The listing builds one solid part. Answer for the finished solid, in the listing's coordinates (mm). A direction names the side the tool comes from. Round coordinates to 2 decimals unless told otherwise and drop trailing zeros. Write each loop counter-clockwise with the first axis right and the second up, starting at its lowest first coordinate (ties: lowest second). Pieces come first, ordered by that corner, then holes.
from build123d import *

# Parameters (mm, degrees)
F1_DEPTH = 6.35
F2_T     = -6.35


with BuildPart() as f1:
    # F0 (on Top) → F1 (new body)
    with BuildSketch(Plane.XY):
        Polygon((38.1, 38.1), (38.1, 76.2), (-38.1, 76.2), (-38.1, 38.1), (-50.8, 38.1), (-50.8, -38.1), (-38.1, -38.1), (-38.1, -76.2), (38.1, -76.2), (38.1, -38.1), (50.8, -38.1), (50.8, 38.1), align=None)
    extrude(amount=F1_DEPTH)

    # F2
    f2_openings = [f1.faces().sort_by_distance(p)[0] for p in [
        (0, 0, 6.35),
        (0, 0, 0),
    ]]
    offset(amount=F2_T, openings=f2_openings, kind=Kind.INTERSECTION)


solid = f1.part
1. Straight lines are drawn through the part: line 1 along X through (y, z) = (-13, 6); line 2 along Y through (x, z) = (-34, 0.75); line 3 along X through (y, z) = (-65.5, 1.5). For each, find the intervals that lie inside material, in ascending order.
Geometry says:
line 1: x = -50.8 to -44.45, 44.45 to 50.8
line 2: y = -76.2 to -31.75, 31.75 to 76.2
line 3: x = -38.1 to -31.75, 31.75 to 38.1
2. Section A-A on y = 34 is taken. Determine the outline of the cut face in (x, z).
Geometry says:
outline: (-50.8, 0) - (-31.75, 0) - (-31.75, 6.35) - (-50.8, 6.35) - close; (31.75, 0) - (50.8, 0) - (50.8, 6.35) - (31.75, 6.35) - close
3. Section C-C on z = 2 is taken. Determine the outline of the cut face in (x, y), plus the area to 3 significant figures.
Geometry says:
outline: (-50.8, -38.1) - (-38.1, -38.1) - (-38.1, -76.2) - (38.1, -76.2) - (38.1, -38.1) - (50.8, -38.1) - (50.8, 38.1) - (38.1, 38.1) - (38.1, 76.2) - (-38.1, 76.2) - (-38.1, 38.1) - (-50.8, 38.1) - close; hole (-44.45, -31.75) - (-31.75, -31.75) - (-31.75, -69.85) - (31.75, -69.85) - (31.75, -31.75) - (44.45, -31.75) - (44.45, 31.75) - (31.75, 31.75) - (31.75, 69.85) - (-31.75, 69.85) - (-31.75, 31.75) - (-44.45, 31.75) - close
area: 3,060 mm2
4. Given pin 1 (1 mm diameter, centred on y = -38.5, z = 1, fed in from +X); pin 2 (3 mm diameter, centred on y = -45.5, z = 3.5, fed in from +X); pin 3 (3 mm diameter, centred on x = -44, z = 3, fed in from +Y); pin 4 (3 mm diameter, centred on y = 65, z = 4, fed in from -X), each flat-ended and moving along its own axis, determine where each tip first touches the part or whether it passes through.
Geometry says:
pin 1: stops at x = 50.8
pin 2: stops at x = 38.1
pin 3: stops at y = 38.1
pin 4: stops at x = -38.1
5. Section B-B on x = 8 is taken. Determine the outline of the cut face in (y, z).
Geometry says:
outline: (-76.2, 0) - (-69.85, 0) - (-69.85, 6.35) - (-76.2, 6.35) - close; (69.85, 0) - (76.2, 0) - (76.2, 6.35) - (69.85, 6.35) - close
6. A tool of negligible diameter and unlimited length cuts with its end or side. For faces 1 (the face through (38.1, 57, 3)), 2 (the face through (-45, -38.1, 3)), 3 (the face through (38.1, -57, 3)), from which of +Z, -Z, +X, -X, +Y, -Y can it reach the whole face along a straight path? Write none if from no direction.
Geometry says:
face 1: +Z, -Z, +X, +Y
face 2: +Z, -Z, -X, -Y
face 3: +Z, -Z, +X, -Y
7. For a pull along X with two mould halves and no side action, classify faces 4 (the face through (-38, 31.75, 3)), 5 (the face through (50.8, -1, 3)), 6 (the face through (-44, 38.1, 3)), 7 (the face through (31.75, 51, 3)) as released by +X, released by -X, zero draft, split by the parting line, or undercut.
Geometry says:
face 4: undercut
face 5: released by +X
face 6: zero draft
face 7: undercut
